The listing builds one solid part. Answer for the finished solid, in the listing's coordinates (mm). Coordinates: 2 decimals unless noted, no trailing zeros. Write each loop counter-clockwise with the first axis right and the second up, starting at its lowest first coordinate (ties: lowest second). Pieces come first, ordered by that corner, then holes.
(1) The part is cut by section A-A on y = -236. Determine the outline of the cut face in (x, z) (3 decimals), plus the area to 3 significant figures.
(2) The part is cut by section B-B on x = 1.3. Give the number of separate pieces and of enclosed holes in the cut face, plus the area to 3 significant figures.
(3) Given P1, Ø1.8, axis at x = 4, z = 54.5, coming from the +Y side, flat-ended and moving along its own axis, determine where the tip first touches the part or whether it passes through.
(4) Straight lines are drawn through the part: line 1 (Z direction, x = 5.2, y = -210.5) (3 decimals); line 2 (Y direction, x = 2.6, z = 39). For each, find the intervals that lie inside material, in ascending order.
Autodesk Inventor part; units mm, degrees
ref_plane "YZ Plane" through (0, 0, 0) normal (1, 0, 0) x (0, 1, 0)
ref_plane "XZ Plane" through (0, 0, 0) normal (0, 1, 0) x (-1, 0, 0)
ref_plane "XY Plane" through (0, 0, 0) normal (0, 0, 1) x (1, 0, 0)
sketch "Sketch1" plane through (0, 0, 0) normal (1, 0, 0) x (0, 1, 0)
  line L0 (0, 70) -> (-341.3, 70)
  line L1 (-341.3, 70) -> (-341.3, 0)
  line L2 (-341.3, 0) -> (0, 0)
  line L3 (0, 0) -> (0, 60) construction
  line L4 (0, 70) -> (6, 70)
  line L5 (6, 70) -> (6, 60)
  line L6 (6, 60) -> (0, 60)
  line L7 (0, 50) -> (6, 50)
  line L8 (6, 50) -> (6, 40)
  line L9 (6, 40) -> (0, 40)
  line L10 (0, 30) -> (6, 30)
  line L11 (6, 30) -> (6, 20)
  line L12 (6, 20) -> (0, 20)
  line L13 (0, 10) -> (6, 10)
  line L14 (6, 10) -> (6, 0)
  line L15 (6, 0) -> (0, 0)
  line L16 (0, 60) -> (0, 50)
  line L17 (0, 40) -> (0, 30)
  line L18 (0, 20) -> (0, 10)
  line L19 (-10.15, 28.525) -> (-19.85, 28.525)
  line L20 (-19.85, 28.525) -> (-19.85, 22.675)
  line L21 (-19.85, 22.675) -> (-10.15, 22.675)
  line L22 (-10.15, 22.675) -> (-10.15, 28.525)
  line L23 (-10, 28.6) -> (-331.3, 28.6) construction
  line L24 (-331.3, 28.6) -> (-331.3, 22.6) construction
  line L25 (-331.3, 22.6) -> (-10, 22.6) construction
  line L26 (-10, 22.6) -> (-10, 28.6) construction
  line L27 (-15, 28.6) -> (-15, 22.6) construction
  line L28 (-30.15, 22.675) -> (-30.15, 28.525)
  line L29 (-30.15, 28.525) -> (-39.85, 28.525)
  line L30 (-39.85, 22.675) -> (-30.15, 22.675)
  line L31 (-39.85, 28.525) -> (-39.85, 22.675)
  line L32 (-50.15, 22.675) -> (-50.15, 28.525)
  line L33 (-50.15, 28.525) -> (-59.85, 28.525)
  line L34 (-59.85, 22.675) -> (-50.15, 22.675)
  line L35 (-59.85, 28.525) -> (-59.85, 22.675)
  line L36 (-70.15, 22.675) -> (-70.15, 28.525)
  line L37 (-70.15, 28.525) -> (-79.85, 28.525)
  line L38 (-79.85, 22.675) -> (-70.15, 22.675)
  line L39 (-79.85, 28.525) -> (-79.85, 22.675)
  line L40 (-90.15, 22.675) -> (-90.15, 28.525)
  line L41 (-90.15, 28.525) -> (-99.85, 28.525)
  line L42 (-99.85, 22.675) -> (-90.15, 22.675)
  line L43 (-99.85, 28.525) -> (-99.85, 22.675)
  line L44 (-110.15, 22.675) -> (-110.15, 28.525)
  line L45 (-110.15, 28.525) -> (-119.85, 28.525)
  line L46 (-119.85, 22.675) -> (-110.15, 22.675)
  line L47 (-119.85, 28.525) -> (-119.85, 22.675)
  line L48 (-130.15, 22.675) -> (-130.15, 28.525)
  line L49 (-130.15, 28.525) -> (-139.85, 28.525)
  line L50 (-139.85, 22.675) -> (-130.15, 22.675)
  line L51 (-139.85, 28.525) -> (-139.85, 22.675)
  line L52 (-150.15, 22.675) -> (-150.15, 28.525)
  line L53 (-150.15, 28.525) -> (-159.85, 28.525)
  line L54 (-159.85, 22.675) -> (-150.15, 22.675)
  line L55 (-159.85, 28.525) -> (-159.85, 22.675)
  line L56 (-170.15, 22.675) -> (-170.15, 28.525)
  line L57 (-170.15, 28.525) -> (-179.85, 28.525)
  line L58 (-179.85, 22.675) -> (-170.15, 22.675)
  line L59 (-179.85, 28.525) -> (-179.85, 22.675)
  line L60 (-190.15, 22.675) -> (-190.15, 28.525)
  line L61 (-190.15, 28.525) -> (-199.85, 28.525)
  line L62 (-199.85, 22.675) -> (-190.15, 22.675)
  line L63 (-199.85, 28.525) -> (-199.85, 22.675)
  line L64 (-210.15, 22.675) -> (-210.15, 28.525)
  line L65 (-210.15, 28.525) -> (-219.85, 28.525)
  line L66 (-219.85, 22.675) -> (-210.15, 22.675)
  line L67 (-219.85, 28.525) -> (-219.85, 22.675)
  line L68 (-230.15, 22.675) -> (-230.15, 28.525)
  line L69 (-230.15, 28.525) -> (-239.85, 28.525)
  line L70 (-239.85, 22.675) -> (-230.15, 22.675)
  line L71 (-239.85, 28.525) -> (-239.85, 22.675)
  line L72 (-250.15, 22.675) -> (-250.15, 28.525)
  line L73 (-250.15, 28.525) -> (-259.85, 28.525)
  line L74 (-259.85, 22.675) -> (-250.15, 22.675)
  line L75 (-259.85, 28.525) -> (-259.85, 22.675)
  line L76 (-270.15, 22.675) -> (-270.15, 28.525)
  line L77 (-270.15, 28.525) -> (-279.85, 28.525)
  line L78 (-279.85, 22.675) -> (-270.15, 22.675)
  line L79 (-279.85, 28.525) -> (-279.85, 22.675)
  line L80 (-290.15, 22.675) -> (-290.15, 28.525)
  line L81 (-290.15, 28.525) -> (-299.85, 28.525)
  line L82 (-299.85, 22.675) -> (-290.15, 22.675)
  line L83 (-299.85, 28.525) -> (-299.85, 22.675)
  line L84 (-310.15, 22.675) -> (-310.15, 28.525)
  line L85 (-310.15, 28.525) -> (-319.85, 28.525)
  line L86 (-319.85, 22.675) -> (-310.15, 22.675)
  line L87 (-319.85, 28.525) -> (-319.85, 22.675)
  point P0 (0, 35)
  point P1 (-170.65, 0)
  point P2 (3, 70)
  point P3 (3, 50)
  point P4 (3, 30)
  point P5 (3, 10)
  point P6 (-10.15, 25.6)
  point P7 (-10, 25.6)
  point P8 (0, 35)
  point P9 (-15, 25.6)
  point P10 (-15, 22.675)
  point P11 (-30.15, 25.6)
  point P12 (-35, 22.675)
  point P13 (-50.15, 25.6)
  point P14 (-55, 22.675)
  point P15 (-70.15, 25.6)
  point P16 (-75, 22.675)
  point P17 (-90.15, 25.6)
  point P18 (-95, 22.675)
  point P19 (-110.15, 25.6)
  point P20 (-115, 22.675)
  point P21 (-130.15, 25.6)
  point P22 (-135, 22.675)
  point P23 (-150.15, 25.6)
  point P24 (-155, 22.675)
  point P25 (-170.15, 25.6)
  point P26 (-175, 22.675)
  point P27 (-190.15, 25.6)
  point P28 (-195, 22.675)
  point P29 (-210.15, 25.6)
  point P30 (-215, 22.675)
  point P31 (-230.15, 25.6)
  point P32 (-235, 22.675)
  point P33 (-250.15, 25.6)
  point P34 (-255, 22.675)
  point P35 (-270.15, 25.6)
  point P36 (-275, 22.675)
  point P37 (-290.15, 25.6)
  point P38 (-295, 22.675)
  point P39 (-310.15, 25.6)
  point P40 (-315, 22.675)
  dimension "d7" = 70
  dimension "d18" = 6
  dimension "d21" = 10
  dimension "d24" = 341.3
  dimension "d35" = 20
  dimension "d49" = 5.85
  dimension "d50" = 9.7
  dimension "d51" = 6
  dimension "d52" = 9.4
  dimension "d53" = 10
  dimension "d58" = 10
  dimension "d60" = 5
  dimension "d63" = 20
extrude "Extrusion1" add sketch "Sketch1" along normal blind 6
fillet "Fillet1" radius 5 2 edges at (3, -341.3, 70) (3, -341.3, 0)
equation "\"d7\" = moduleMountH"
equation "\"d18\" = fingerH"
equation "\"d21\" = fingerW"
equation "\"d24\" = supportL"
equation "\"d35\" = fingerSpacing"
equation "\"d49\" = fingerholeH"
equation "\"d51\" = thickness"
equation "\"d58\" = 0.5 * fingerSpacing"
equation "\"d63\" = fingerSpacing"
equation "\"d44\" = thickness"
equation "\"d73\" = supportsFilletR"
equation "\"moduleWidth\" = 118"
equation "\"moduleHeight\" = 96"
equation "\"moduleMountH\" = 70"
equation "\"moduleMountD\" = 6.8"
equation "\"moduleCornerR\" = 5"
equation "\"d4\" = moduleCornerR"
equation "\"d5\" = moduleMountD"
equation "\"d6\" = moduleMountD"
equation "\"d8\" = moduleMountD"
equation "\"d10\" = moduleMountD"
equation "\"moduleOpeningR\" = 25"
equation "\"d13\" = moduleOpeningR"
equation "\"thickness\" = 6"
equation "\"d15\" = thickness"
equation "\"d16\" = 0"
equation "\"kerf\" = 0.15"
equation "\"fingerW\" = 10"
equation "\"fingerSpacing\" = 20"
equation "\"fingerholeW\" = fingerW - 2 * kerf"
equation "\"fingerholeH\" = thickness - kerf"
equation "\"moduleMountClearance\" = 19"
equation "\"actuatorW\" = 28"
equation "\"actuatorH\" = 40.8"
equation "\"openingMFC\" = 45"
equation "\"d28\" = thickness"
equation "\"d29\" = thickness"
equation "\"d30\" = 0.5 * actuatorH + thickness"
equation "\"d31\" = 15"
equation "\"d32\" = fingerholeH"
equation "\"d33\" = fingerholeW"
equation "\"d41\" = fingerholeH"
equation "\"d42\" = fingerholeW"
equation "\"chairThickness\" = 12.7"
equation "\"supportL\" = -chairThickness + dildoL + actuatorMountL - thickness"
equation "\"d0\" = moduleHeight"
equation "\"d1\" = moduleWidth"
equation "\"d17\" = openingMFC"
equation "\"d19\" = moduleMountClearance"
equation "\"fingerH\" = thickness"
equation "\"supportSpacingFromMounting\" = 15"
equation "\"d54\" = fingerholeH"
equation "\"d55\" = fingerholeW"
equation "\"d64\" = 9.4"
equation "\"supportsCTCZ\" = d64"
equation "\"supportXW\" = -2 * thickness + moduleMountW - 2 * supportSpacingFromMounting + kerf"
equation "\"supportsFilletR\" = 5"
properties part number "Module_supportZ_MFC"
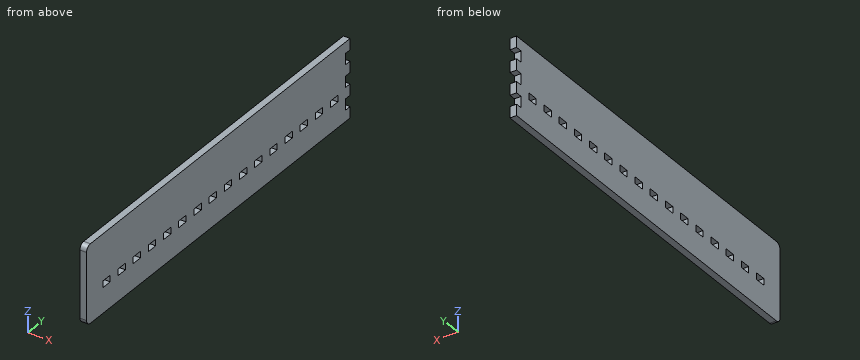
Model answer:
1. outline: (0, 0) - (6, 0) - (6, 22.675) - (0, 22.675) - close; (0, 28.525) - (6, 28.525) - (6, 70) - (0, 70) - close
1. area: 385 mm2
2. separate pieces: 1
2. enclosed holes: 16
2. area: 23,200 mm2
3. P1: stops at y = 0
4. line 1: z = 0 to 22.675, 28.525 to 70
4. line 2: y = -341.3 to 0
